Geometry: final body of the model. Coordinates: model frame, mm. Give positions to 0.01 mm unless a question says otherwise; leave off trailing zeros. Loops run counter-clockwise (first coordinate to the right, second up) from the corner with the lowest first, then second, coordinate; pieces in that order, holes last. Notation, with made-up numbers: M -23.5,-31 L -0.5,-31 A17 ccw -0.5,-20 Z; hole C 36,76.25 d2. An arc over 180 degrees is marked long. Put each result on its own line as item: value.
```python
from build123d import *

# Parameters (mm, degrees)
F0_R     = 75
F0_R_2   = 2.5
F0_R_3   = 10.5
F1_DEPTH = 10
F2_R     = 5
F3_R     = 75
F3_R_2   = 2.5
F4_DEPTH = 9
F5_SIZE  = 8.99999


# Not quite as in the source:
# - a fillet or chamfer is up to 0.001 mm smaller than in the source, because OpenCascade refuses the exact size


with BuildPart() as f1:
    # F0 (on Top) → F1 (new body)
    with BuildSketch(Plane.XY):
        Circle(F0_R)
        with Locations((-35, -60.6217782649)):
            Circle(F0_R_2, mode=Mode.SUBTRACT)
        with Locations((-60.6217782649, -35)):
            Circle(F0_R_2, mode=Mode.SUBTRACT)
        with BuildLine():
            ThreePointArc((-5, -54.7722557505), (-38.8908729653, -38.8908729653), (-54.7722557505, -5))
            Line((-54.7722557505, -5), (-19.364916731, -5))
            ThreePointArc((-19.364916731, -5), (-14.1421356237, -14.1421356237), (-5, -19.364916731))
            Line((-5, -19.364916731), (-5, -54.7722557505))
        make_face(mode=Mode.SUBTRACT)
        with Locations((0, -70)):
            Circle(F0_R_2, mode=Mode.SUBTRACT)
        with Locations((35, -60.6217782649)):
            Circle(F0_R_2, mode=Mode.SUBTRACT)
        with BuildLine():
            Line((19.364916731, -5), (54.7722557505, -5))
            ThreePointArc((54.7722557505, -5), (38.8908729653, -38.8908729653), (5, -54.7722557505))
            Line((5, -54.7722557505), (5, -19.364916731))
            ThreePointArc((5, -19.364916731), (14.1421356237, -14.1421356237), (19.364916731, -5))
        make_face(mode=Mode.SUBTRACT)
        with Locations((60.6217782649, -35)):
            Circle(F0_R_2, mode=Mode.SUBTRACT)
        with Locations((-70, 0)):
            Circle(F0_R_2, mode=Mode.SUBTRACT)
        with Locations((-60.6217782649, 35)):
            Circle(F0_R_2, mode=Mode.SUBTRACT)
        with BuildLine():
            Line((-5, 54.7722557505), (-5, 19.364916731))
            ThreePointArc((-5, 19.364916731), (-14.1421356237, 14.1421356237), (-19.364916731, 5))
            Line((-19.364916731, 5), (-54.7722557505, 5))
            ThreePointArc((-54.7722557505, 5), (-38.8908729653, 38.8908729653), (-5, 54.7722557505))
        make_face(mode=Mode.SUBTRACT)
        with Locations((-35, 60.6217782649)):
            Circle(F0_R_2, mode=Mode.SUBTRACT)
        Circle(F0_R_3, mode=Mode.SUBTRACT)
        with BuildLine():
            ThreePointArc((5, 54.7722557505), (38.8908729653, 38.8908729653), (54.7722557505, 5))
            Line((54.7722557505, 5), (19.364916731, 5))
            ThreePointArc((19.364916731, 5), (14.1421356237, 14.1421356237), (5, 19.364916731))
            Line((5, 19.364916731), (5, 54.7722557505))
        make_face(mode=Mode.SUBTRACT)
        with Locations((70, 0)):
            Circle(F0_R_2, mode=Mode.SUBTRACT)
        with Locations((60.6217782649, 35)):
            Circle(F0_R_2, mode=Mode.SUBTRACT)
        with Locations((0, 70)):
            Circle(F0_R_2, mode=Mode.SUBTRACT)
        with Locations((35, 60.6217782649)):
            Circle(F0_R_2, mode=Mode.SUBTRACT)
    extrude(amount=F1_DEPTH)

    # F2
    f2_edges = [f1.edges().sort_by_distance(p)[0] for p in [
        (5, -54.772256, 5),
        (5, -19.364917, 5),
        (19.364917, -5, 5),
        (19.364917, 5, 5),
        (5, 19.364917, 5),
        (-5, 19.364917, 5),
        (-19.364917, 5, 5),
        (-5, -19.364917, 5),
        (-19.364917, -5, 5),
        (54.772256, 5, 5),
        (54.772256, -5, 5),
        (5, 54.772256, 5),
        (-54.772256, -5, 5),
        (-5, 54.772256, 5),
        (-5, -54.772256, 5),
        (-54.772256, 5, 5),
    ]]
    fillet(f2_edges, radius=F2_R)

    # F3 (on face) → F4 (join)
    with BuildSketch(Plane.XY.offset(10)):
        Circle(F3_R)
        with Locations((-35, -60.6217782649)):
            Circle(F3_R_2, mode=Mode.SUBTRACT)
        with Locations((-60.6217782649, -35)):
            Circle(F3_R_2, mode=Mode.SUBTRACT)
        with Locations((0, -70)):
            Circle(F3_R_2, mode=Mode.SUBTRACT)
        with Locations((35, -60.6217782649)):
            Circle(F3_R_2, mode=Mode.SUBTRACT)
        with Locations((60.6217782649, -35)):
            Circle(F3_R_2, mode=Mode.SUBTRACT)
        with Locations((-70, 0)):
            Circle(F3_R_2, mode=Mode.SUBTRACT)
        with Locations((-60.6217782649, 35)):
            Circle(F3_R_2, mode=Mode.SUBTRACT)
        with Locations((-35, 60.6217782649)):
            Circle(F3_R_2, mode=Mode.SUBTRACT)
        with BuildLine():
            ThreePointArc((53.8887743412, 11), (54.7214884153, 5.5279929103), (55, 0))
            ThreePointArc((55, 0), (54.7214884153, -5.5279929103), (53.8887743412, -11))
            ThreePointArc((53.8887743412, -11), (38.8908729653, -38.8908729653), (11, -53.8887743412))
            ThreePointArc((11, -53.8887743412), (0, -55), (-11, -53.8887743412))
            ThreePointArc((-11, -53.8887743412), (-38.8908729653, -38.8908729653), (-53.8887743412, -11))
            ThreePointArc((-53.8887743412, -11), (-55, 0), (-53.8887743412, 11))
            ThreePointArc((-53.8887743412, 11), (-38.8908729653, 38.8908729653), (-11, 53.8887743412))
            ThreePointArc((-11, 53.8887743412), (0, 55), (11, 53.8887743412))
            ThreePointArc((11, 53.8887743412), (38.8908729653, 38.8908729653), (53.8887743412, 11))
        make_face(mode=Mode.SUBTRACT)
        with Locations((70, 0)):
            Circle(F3_R_2, mode=Mode.SUBTRACT)
        with Locations((60.6217782649, 35)):
            Circle(F3_R_2, mode=Mode.SUBTRACT)
        with Locations((0, 70)):
            Circle(F3_R_2, mode=Mode.SUBTRACT)
        with Locations((35, 60.6217782649)):
            Circle(F3_R_2, mode=Mode.SUBTRACT)
    extrude(amount=F4_DEPTH)

    # F5 (size 9 in the source; OpenCascade refuses exactly that, so slightly less here)
    f5_edges = [f1.edges().sort_by_distance(p)[0] for p in [
        (53.888774, 11, 19),
    ]]
    chamfer(f5_edges, length=F5_SIZE)


solid = f1.part
```
Item 1: Pin query (flat end, axial travel): pin 1 Ø5 at (y, z) = (-33, 7.5) entering from -X; pin 2 Ø24 at (x, y) = (0, 0) entering from +Z; pin 3 Ø10 at (y, z) = (0.5, 2.5) entering from -X; pin 4 Ø1.5 at (x, z) = (10, 7.5) entering from +Y. Return the tip coordinate at first contact, or that it passes through.
Output values:
pin 1: x = -68.52
pin 2: z = 10
pin 3: x = -75
pin 4: y = 74.43
Item 2: Section A-A on x = 0. Count the separate pieces of the cut face and the enclosed holes in it, then the cut area to 3 significant figures.
Output values:
separate pieces: 4
enclosed holes: 0
area: 1,380 mm²
Item 3: Section B-B on y = -70. Output: boundary loops of the cut face in (x, z).
Output values:
outline: M -26.93,0 L -2.5,0 L -2.5,19 L -26.93,19 Z; M 2.5,0 L 26.93,0 L 26.93,19 L 2.5,19 Z
Item 4: Mould query, pull axis X, two halves, no side actions, for faces 1 (the cylindrical face through (-9.764, 74.362, 9.367)), 2 (the flat face through (5, -36, 5)). Classes: pulls with the +X half, pulls with the -X half, needs draft (parallel to the pull), parting line crosses it, or undercut.
Output values:
face 1: parting line crosses it
face 2: undercut
Item 5: Line query: probe 1 along Y at (x, z) = (0, 13.25); probe 2 along X at (y, z) = (18, 7.75); probe 3 along Y at (x, z) = (16.5, 1.25). Output: solid intervals per line, ascending. Write a range as [from, to].
Output values:
probe 1: [-75, -72.5], [-67.5, -58.25], [58.25, 67.5], [72.5, 75]
probe 2: [-72.81, -51.97], [-8.72, 8.72], [51.97, 72.81]
probe 3: [-73.16, -52.47], [-11.3, 11.3], [52.47, 73.16]
